Here's the drawing with two shaded views (mm, measured from the low corner). I have some questions. Coordinates: 2 decimals unless noted, no trailing zeros. Order: outer loops, then holes, each group sorted by start corner. A loop starts at its lowest first (then second) coordinate and runs counter-clockwise, first axis right, second up. Notation, with made-up numbers: (-16, 79.25) -> (21, 79.25) arc R29 cw to (21, 99.25) -> close; hole circle Ø8 at (73, 41.5). An arc over 180 degrees is marked (long way). Write item = value, one per line.
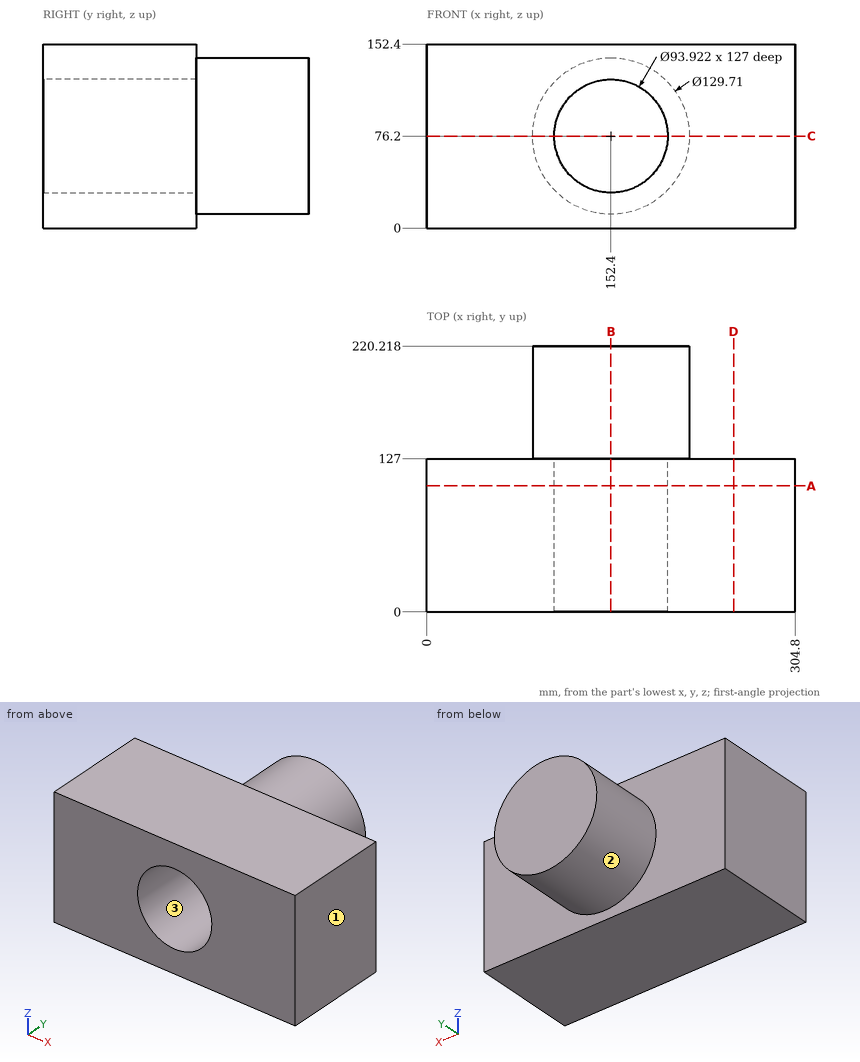
Item 1: I want a section at A-A, the plane y = 104.5. Please give me the cut outline in (x, z), plus the area to 3 significant figures.
A:
outline = (0, 0) -> (304.8, 0) -> (304.8, 152.4) -> (0, 152.4) -> close; hole circle Ø93.92 at (152.4, 76.2)
area = 39,500 mm2
Item 2: I want a section at D-D, the plane x = 254. Please give me the cut outline in (y, z).
A:
outline = (0, 0) -> (127, 0) -> (127, 152.4) -> (0, 152.4) -> close
Item 3: If we mould it in two halves opening along Z, with no side actions, what happens to the marked faces 1, 2 and 3? For each: pulls with the +Z half, pulls with the -Z half, needs draft (parallel to the pull), parting line crosses it, or undercut.
A:
face_1 = needs draft
face_2 = parting line crosses it
face_3 = undercut
Item 4: If I drill on probe 1 along Z at (x, y) = (152, 72); probe 2 along X at (y, z) = (73.5, 76.2); probe 3 along Y at (x, z) = (100.5, 22), over which ranges is the centre line in solid material (lowest first)?
A:
probe_1 = 0 to 29.24, 123.16 to 152.4
probe_2 = 0 to 105.44, 199.36 to 304.8
probe_3 = 0 to 127
Item 5: I want a section at C-C, the plane z = 76.2. Please give me the cut outline in (x, y) (1 decimal), plus the area to 3 significant figures.
A:
outline = (0, 0) -> (105.4, 0) -> (105.4, 127) -> (199.4, 127) -> (199.4, 0) -> (304.8, 0) -> (304.8, 127) -> (217.3, 127) -> (217.3, 220.2) -> (87.5, 220.2) -> (87.5, 127) -> (0, 127) -> close
area = 38,900 mm2
Item 6: I'm going to push flat-ended pins straight in: P1, Ø6, axis at y = 193, z = 17.5, coming from the -X side; P2, Ø5, axis at y = 159, z = 20, coming from the +X side (1 decimal); P3, Ø6, axis at y = 169.5, z = 32, coming from the +X side. Where does each tip first touch, or does it pass through?
A:
P1 = 119.18
P2 = 188.8
P3 = 202.49
Item 7: I want a section at B-B, the plane x = 152.4. Please give me the cut outline in (y, z) (1 decimal).
A:
outline = (0, 0) -> (127, 0) -> (127, 11.3) -> (220.2, 11.3) -> (220.2, 141.1) -> (127, 141.1) -> (127, 152.4) -> (0, 152.4) -> (0, 123.2) -> (127, 123.2) -> (127, 29.2) -> (0, 29.2) -> close
